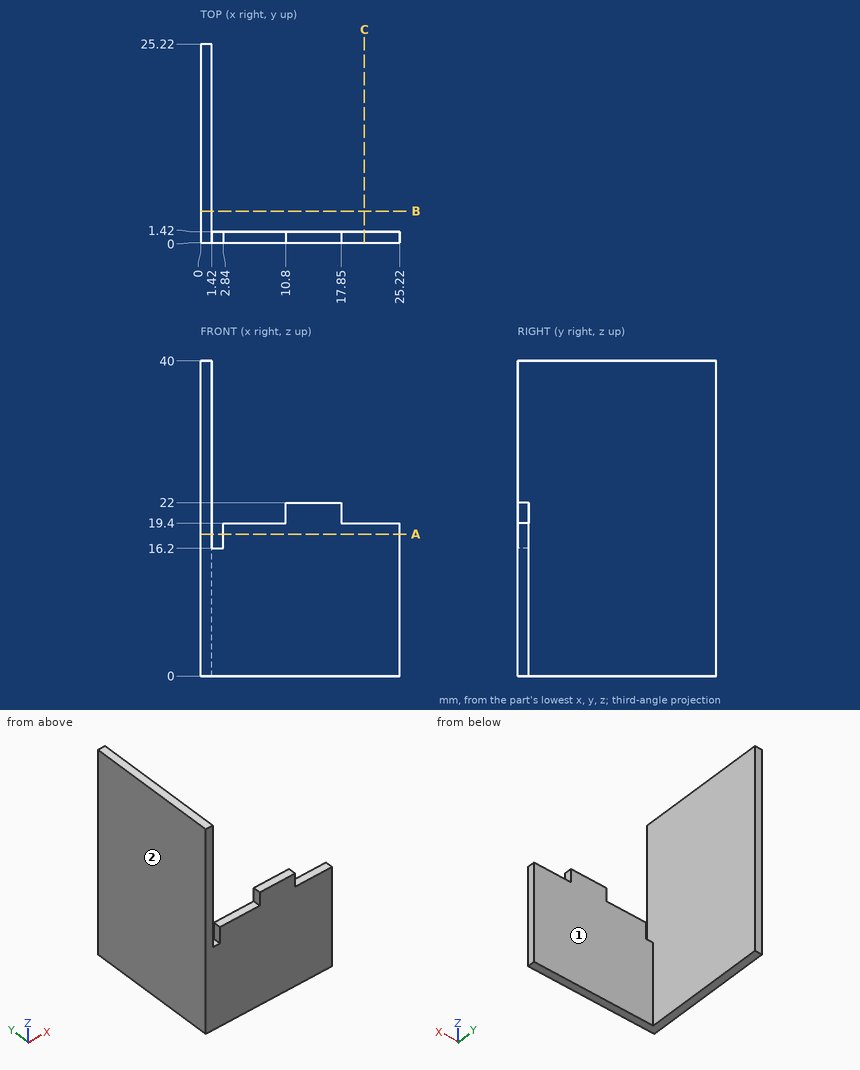
Can you work these out from the drawing? Everything is in mm from the part's minimum corner. A direction names the side the tool comes from. Round coordinates to 2 decimals unless told otherwise and drop trailing zeros. Order: outer loops, then holes, each group sorted by start corner. A loop starts at its lowest first (then second) coordinate and runs counter-clockwise, first axis right, second up.
(1) If we section it at B-B (y = 4): Please give me the cut outline in (x, z), plus the area to 3 significant figures.
Results are:
outline: (0, 0) - (1.42, 0) - (1.42, 40) - (0, 40) - close
area: 56.8 mm2
(2) If we section it at C-C (x = 20.75): Please give me the cut outline in (y, z), plus the area to 3 significant figures.
Results are:
outline: (0, 0) - (1.42, 0) - (1.42, 19.4) - (0, 19.4) - close
area: 27.5 mm2
(3) I'm going to push flat-ended pins straight in: pin 1 (5 mm diameter, centred on y = 22.5, z = 29.5, fed in from +X); pin 2 (8 mm diameter, centred on y = 16, z = 35.5, fed in from -X); pin 3 (1.6 mm diameter, centred on x = 5.5, y = 1, fed in from +Z); pin 4 (6.5 mm diameter, centred on x = 16, z = 7, fed in from +Y). Where does each tip first touch, or does it pass through?
Results are:
pin 1: stops at x = 1.42
pin 2: stops at x = 0
pin 3: stops at z = 19.4
pin 4: stops at y = 1.42
(4) If I drill on L1, parallel to X at y = 11, z = 7.5, over which ranges is the centre line in solid material (lowest first)?
Results are:
L1: x = 0 to 1.42
(5) On a 3-axis mill with a long thin cutter (end or side, diameter ignored), from which of +Z, -Z, +X, -X, +Y, -Y can I reach the whole of each face in a straight line? I mean the marked faces 1 and 2. Say none if no direction works.
Results are:
face 1: +Z, -Z, +X, +Y
face 2: +Z, -Z, -X, +Y, -Y
(6) If we section it at A-A (z = 18): Please give me the cut outline in (x, y).
Results are:
outline: (0, 0) - (1.42, 0) - (1.42, 25.22) - (0, 25.22) - close; (2.84, 0) - (25.22, 0) - (25.22, 1.42) - (2.84, 1.42) - close
